Part model, mm, in its own coordinate system. A direction names the side the tool comes from. Round coordinates to 2 decimals unless told otherwise and drop trailing zeros. Loops run counter-clockwise (first coordinate to the right, second up) from the corner with the lowest first, then second, coordinate; pieces in that order, holes last. Notation, with made-up numbers: (-25.75, 0.5) -> (-19.75, 0.5) arc R28 ccw to (-19.75, 37.5) -> close; hole circle Ø6 at (71, -36). An arc over 180 degrees is marked (long way). Answer as CSV lines item,"result".
from build123d import *

# Parameters (mm, degrees)
F1_DEPTH = 19.05
F3_DEPTH = 12.7
F4_W     = 16.968144
F4_H     = 30.109933
F5_DEPTH = 25.4


with BuildPart() as f1:
    # F0 (on Top) → F1 (new body)
    with BuildSketch(Plane.XY):
        with BuildLine():
            Line((33.250909, -20.666365), (33.250909, 20.666365))
            Line((33.250909, 20.666365), (-33.250909, 20.666365))
            Line((-33.250909, 20.666365), (-33.250909, -20.666365))
            ThreePointArc((-33.250909, -20.666365), (0, -39.149988), (33.250909, -20.666365))
        make_face()
    extrude(amount=F1_DEPTH)

    # F2 (on face) → F3 (join)
    with BuildSketch(Plane(origin=(0, 20.666365, 0), x_dir=(-1, 0, 0), z_dir=(0, 1, 0))):
        with BuildLine():
            Line((-33.250909, 19.05), (-33.250909, 0))
            Line((-33.250909, 0), (33.250909, 0))
            Line((33.250909, 0), (33.250909, 19.05))
            Line((33.250909, 19.05), (33.250909, 79.54818))
            Line((33.250909, 79.54818), (8.83812, 79.54818))
            Line((8.83812, 79.54818), (8.83812, 46.779379))
            ThreePointArc((8.83812, 46.779379), (0, 37.941259), (-8.83812, 46.779379))
            Line((-8.83812, 46.779379), (-8.83812, 79.54818))
            Line((-8.83812, 79.54818), (-15.810801, 79.54818))
            Line((-15.810801, 79.54818), (-33.250909, 79.54818))
            Line((-33.250909, 79.54818), (-33.250909, 19.05))
        make_face()
    extrude(amount=F3_DEPTH)

    # F4 (on face) → F5 (cut)
    with BuildSketch(Plane(origin=(0, 33.366365, 0), x_dir=(-1, 0, 0), z_dir=(0, 1, 0))):
        with Locations((-24.766837, 15.054966)):
            Rectangle(F4_W, F4_H)
    extrude(amount=-F5_DEPTH, mode=Mode.SUBTRACT)


solid = f1.part
Q1. Drill centre lines: line 1 along X through (y, z) = (26.5, 59); line 2 along X through (y, z) = (8.5, 18.5); line 3 along Z through (x, y) = (-17, -17). Where is each one in solid material? Low to high.
Geometry results:
line 1,"-33.25 to -8.84, 8.84 to 33.25"
line 2,"-33.25 to 16.28"
line 3,"0 to 19.05"
Q2. Saw through at B-B, the plane x = 0. Write the cut outline in (y, z), then the cut area to 3 significant figures.
Geometry results:
outline,"(-39.15, 0) -> (33.37, 0) -> (33.37, 37.94) -> (20.67, 37.94) -> (20.67, 19.05) -> (-39.15, 19.05) -> close"
area,"1,620 mm2"
Q3. Which spindle directions (+Z, -Z, +X, -X, +Y, -Y) get a long thin tool onto all of the face, cutting with end or side? Do faces 4 (the face through (8.838, 27, 63)), 5 (the face through (0, -9, 19.05)), 6 (the face through (16.283, 21, 11)). Say none if no direction does.
Geometry results:
face 4,"+Z, +Y, -Y"
face 5,"+Z, +X, -X, -Y"
face 6,"-Z, +X, +Y"
Q4. Saw through at D-D, the plane x = 22. Write the cut outline in (y, z).
Geometry results:
outline,"(-32.38, 0) -> (7.97, 0) -> (7.97, 19.05) -> (-32.38, 19.05) -> close; (20.67, 30.11) -> (33.37, 30.11) -> (33.37, 79.55) -> (20.67, 79.55) -> close"
Q5. Saw through at C-C, the plane y = 26. Write the cut outline in (x, z).
Geometry results:
outline,"(-33.25, 0) -> (16.28, 0) -> (16.28, 30.11) -> (33.25, 30.11) -> (33.25, 79.55) -> (8.84, 79.55) -> (8.84, 46.78) arc R8.84 cw to (-8.84, 46.78) -> (-8.84, 79.55) -> (-33.25, 79.55) -> close"
Q6. Drop flat-ended pins along their axis: P1, Ø4, axis at x = 27, y = 29, coming from the -Z side; P2, Ø18, axis at x = 15, y = 4.5, coming from the +Z side; P3, Ø12.5, axis at y = 21, z = 8.5, coming from the +X side. Give the stop position or say it passes through.
Geometry results:
P1,"z = 30.11"
P2,"z = 19.05"
P3,"x = 16.28"
Q7. Saw through at A-A, the plane z = 66.5. Write the cut outline in (x, y), then the cut area to 3 significant figures.
Geometry results:
outline,"(-33.25, 20.67) -> (-8.84, 20.67) -> (-8.84, 33.37) -> (-33.25, 33.37) -> close; (8.84, 20.67) -> (33.25, 20.67) -> (33.25, 33.37) -> (8.84, 33.37) -> close"
area,"620 mm2"
Q8. Two-plate mould, pull along X, no slides. Class faces 1 (the face through (-33.251, 24, 22)), 2 (the face through (-0.194, 26.927, 37.943)), 3 (the face through (33.251, 27, 55)): pulls with the +X half, pulls with the -X half, needs draft (parallel to the pull), parting line crosses it, or undercut.
Geometry results:
face 1,"pulls with the -X half"
face 2,"undercut"
face 3,"pulls with the +X half"
